Source: CAD feature listing. Evaluate the final solid. Frame: model axes, mm. Coordinates: 2 decimals unless noted, no trailing zeros. Write each loop counter-clockwise with the first axis right and the second up, starting at its lowest first coordinate (ties: lowest second). Pieces come first, ordered by that corner, then holes. Notation, with made-up numbers: (16, 11) -> (31, 11) arc R24 cw to (31, 46) -> close; hole circle Ø6 at (-21.75, 15). An arc over 180 degrees is marked (long way). One line per item, written item: value. Start each with the question number.
1. Line query: line 1 (X direction, y = -2, z = 62); line 2 (Y direction, x = 0, z = 34.5); line 3 (Y direction, x = 0, z = 46.5). Output: solid intervals per line, ascending.
2. First-contact query: P1, Ø2, axis at x = -4.5, z = 43.5, coming from the +Y side; P2, Ø10, axis at x = -8.5, z = 24.5, coming from the -Y side. Flat tips, straight axial feed; report the tip coordinate or a pass-through.
3. Section query B-B, the plane y = 3. Output: boundary loops of the cut face in (x, z).
4. Mould query, pull axis Y, two halves, no side actions, for faces 1 (the cylindrical face through (1.08, 4.88, 40.56)), 2 (the flat face through (15, 19, 39)), 3 (the cylindrical face through (0, -15, 39)), 4 (the flat face through (0, 50, 5)). Classes: released by +Y, released by -Y, zero draft, split by the parting line, or undercut.
5. Section query A-A, the plane x = 0. Output: boundary loops of the cut face in (y, z).
6. Section query D-D, the plane y = 41. Output: boundary loops of the cut face in (x, z), and give its area (3 significant figures).
7. Section query C-C, the plane z = 40. Output: boundary loops of the cut face in (x, y).
from build123d import *

# Parameters (mm, degrees)
F1_DEPTH = 80
F3_DEPTH = 55
F5_D     = 10


with BuildPart() as f1:
    # F0 (on Top) → F1 (new body)
    with BuildSketch(Plane.XY):
        with BuildLine():
            ThreePointArc((-15, 0), (0, -15), (15, 0))
            ThreePointArc((15, 0), (0, 15), (-15, 0))
        make_face()
        with BuildLine():
            ThreePointArc((-15, 0), (0, 15), (15, 0))
            Line((15, 0), (15, 50))
            Line((15, 50), (-15, 50))
            Line((-15, 50), (-15, 0))
        make_face()
    extrude(amount=F1_DEPTH)

    # F2 (on face) → F3 (cut)
    with BuildSketch(Plane(origin=(-15, 0, 0), x_dir=(0, -1, 0), z_dir=(-1, 0, 0))):
        with BuildLine():
            ThreePointArc((-50, 9.274351), (-19.274351, 40), (-50, 70.725649))
            Line((-50, 70.725649), (-50, 9.274351))
        make_face()
    extrude(amount=-F3_DEPTH, mode=Mode.SUBTRACT)

    # F5 (through all)
    with Locations(Plane(origin=(0, 0, 0), x_dir=(1, 0, 0), z_dir=(0, 0, -1))):
        with Locations((0, 0)):
            Hole(F5_D / 2)


solid = f1.part
Computed values:
1. line 1: x = -14.87 to -4.58, 4.58 to 14.87
1. line 2: y = -15 to -5, 5 to 19.77
1. line 3: y = -15 to -5, 5 to 19.97
2. P1: stops at y = 19.61
2. P2: stops at y = -14.59
3. outline: (-15, 0) -> (-4, 0) -> (-4, 80) -> (-15, 80) -> close; (4, 0) -> (15, 0) -> (15, 80) -> (4, 80) -> close
4. face 1: undercut
4. face 2: zero draft
4. face 3: released by -Y
4. face 4: released by +Y
5. outline: (-15, 0) -> (-5, 0) -> (-5, 80) -> (-15, 80) -> close; (5, 0) -> (50, 0) -> (50, 9.27) arc R30.73 cw to (50, 70.73) -> (50, 80) -> (5, 80) -> close
6. outline: (-15, 0) -> (15, 0) -> (15, 10.62) -> (-15, 10.62) -> close; (-15, 69.38) -> (15, 69.38) -> (15, 80) -> (-15, 80) -> close
6. area: 637 mm²
7. outline: (-15, 0) arc R15 ccw to (15, 0) -> (15, 19.27) -> (-15, 19.27) -> close; hole circle Ø10 at (0, 0)
